Source: CAD feature listing. Evaluate the final solid. Frame: model axes, mm. Face numbers are marked on the shaded views. A direction names the side the tool comes from. Give positions to 0.01 mm unless a question says otherwise; leave off trailing zeros. Loops run counter-clockwise (first coordinate to the right, second up) from the corner with the lowest first, then second, coordinate; pieces in that order, holes last.
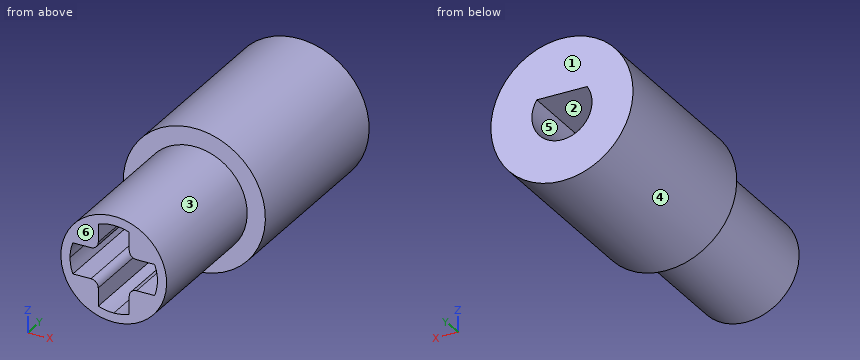
from build123d import *

# Parameters (mm, degrees)
SCHNITT_LINEAR_AUSTRAGEN1_DEPTH = 8
SCHNITT_LINEAR_AUSTRAGEN2_DEPTH = 10


with BuildPart() as part:
    # Skizze1 → Rotation1 (revolve)
    with BuildSketch(Plane.XY, mode=Mode.PRIVATE) as rotation1_sk:
        Polygon((0, 0), (-2.9, 0), (-2.9, 8), (-3.9, 8), (-3.9, 18.3), (0, 18.3), align=None)
    revolve(rotation1_sk.sketch.rotate(Axis((0, 0, 0), (0, 1, 0)), 270), axis=Axis((0, 0, 0), (0, 1, 0)))

    # Skizze3 → Schnitt-Linear austragen1 (cut)
    with BuildSketch(Plane.XZ):
        with BuildLine():
            Line((0.85, 2.244437569), (0.85, 1.25))
            ThreePointArc((0.85, 1.25), (0.967157288, 0.967157288), (1.25, 0.85))
            Line((1.25, 0.85), (2.244437569, 0.85))
            ThreePointArc((2.244437569, 0.85), (2.36078908, 0.432058928), (2.4, 0))
            ThreePointArc((2.4, 0), (2.36078908, -0.432058928), (2.244437569, -0.85))
            Line((2.244437569, -0.85), (1.25, -0.85))
            ThreePointArc((1.25, -0.85), (0.967157288, -0.967157288), (0.85, -1.25))
            Line((0.85, -1.25), (0.85, -2.244437569))
            ThreePointArc((0.85, -2.244437569), (0.432058928, -2.36078908), (0, -2.4))
            ThreePointArc((0, -2.4), (-0.432058928, -2.36078908), (-0.85, -2.244437569))
            Line((-0.85, -2.244437569), (-0.85, -1.25))
            ThreePointArc((-0.85, -1.25), (-0.967157288, -0.967157288), (-1.25, -0.85))
            Line((-1.25, -0.85), (-2.244437569, -0.85))
            ThreePointArc((-2.244437569, -0.85), (-2.36078908, -0.432058928), (-2.4, 0))
            ThreePointArc((-2.4, 0), (-2.36078908, 0.432058928), (-2.244437569, 0.85))
            Line((-2.244437569, 0.85), (-1.25, 0.85))
            ThreePointArc((-1.25, 0.85), (-0.967157288, 0.967157288), (-0.85, 1.25))
            Line((-0.85, 1.25), (-0.85, 2.244437569))
            ThreePointArc((-0.85, 2.244437569), (-0.432058928, 2.36078908), (0, 2.4))
            ThreePointArc((0, 2.4), (0.432058928, 2.36078908), (0.85, 2.244437569))
        make_face()
    extrude(amount=-SCHNITT_LINEAR_AUSTRAGEN1_DEPTH, mode=Mode.SUBTRACT)

    # Skizze4 → Schnitt-Linear austragen2 (cut)
    with BuildSketch(Plane(origin=(0, 18.3, 0), x_dir=(1, 0, 0), z_dir=(0, 1, 0))):
        with BuildLine():
            Line((-1.382931669, -0.9), (1.382931669, -0.9))
            ThreePointArc((1.382931669, -0.9), (0, 1.65), (-1.382931669, -0.9))
        make_face()
    extrude(amount=-SCHNITT_LINEAR_AUSTRAGEN2_DEPTH, mode=Mode.SUBTRACT)


solid = part.part
1) Cut plane A-A (y = 7). Return loops of the section in (x, z), and give its area (3 significant figures).
Checks:
outline: circle Ø5.8 at (0, 0); hole (-2.24, -0.85) - (-1.25, -0.85) arc R0.4 cw to (-0.85, -1.25) - (-0.85, -2.24) arc R2.4 ccw to (0.85, -2.24) - (0.85, -1.25) arc R0.4 cw to (1.25, -0.85) - (2.24, -0.85) arc R2.4 ccw to (2.24, 0.85) - (1.25, 0.85) arc R0.4 cw to (0.85, 1.25) - (0.85, 2.24) arc R2.4 ccw to (-0.85, 2.24) - (-0.85, 1.25) arc R0.4 cw to (-1.25, 0.85) - (-2.24, 0.85) arc R2.4 ccw to start
area: 13.2 mm2
2) Cut plane B-B (x = -0.5). Return loops of the section in (y, z).
Checks:
outline: (0, -2.86) - (8, -2.86) - (8, -3.87) - (18.3, -3.87) - (18.3, -1.57) - (8.3, -1.57) - (8.3, 0.9) - (18.3, 0.9) - (18.3, 3.87) - (8, 3.87) - (8, 2.86) - (0, 2.86) - (0, 2.35) - (8, 2.35) - (8, -2.35) - (0, -2.35) - close
3) Pull-direction query (Z, two-part tool) for the marked faces 4, 5 and 6; classes: released by +Z, released by -Z, zero draft, split by the parting line, or undercut.
Checks:
face 4: split by the parting line
face 5: undercut
face 6: zero draft
4) Ray query, probe 1 along X at (y, z) = (13.75, 0); probe 2 along Y at (x, z) = (0, 0.25); probe 3 along X at (y, z) = (2.25, 1.5). Return the intervals inside material, ascending.
Checks:
probe 1: x = -3.9 to -1.65, 1.65 to 3.9
probe 2: y = 8 to 8.3
probe 3: x = -2.48 to -0.85, 0.85 to 2.48
5) Reachability of the marked faces 1, 2 and 3 from +Z, -Z, +X, -X, +Y, -Y: full face, straight path, thin tool, end or side. Return the list, or none.
Checks:
face 1: +Z, -Z, +X, -X, +Y
face 2: +Y
face 3: -Y
6) Cut plane C-C (y = 11). Return loops of the section in (x, z), and give its area (3 significant figures).
Checks:
outline: circle Ø7.8 at (0, 0); hole (-1.38, 0.9) arc R1.65 ccw (long way) to (1.38, 0.9) - close
area: 40.7 mm2
7) Contact query for flat-ended pins moving along their axis: P1, Ø1.1, axis at y = 5, z = -1.5, coming from the -X side; P2, Ø0.5, axis at x = -1.5, y = 3, coming from the -Z side; P3, Ø0.8, axis at y = 4.5, z = 2, coming from the +X side. Output: stop coordinate, or through.
Checks:
P1: stops at x = -2.74
P2: stops at z = -2.62
P3: stops at x = 2.42
